from build123d import *

# Parameters (mm, degrees)
SKETCH_1_R          = 19.05
EXTRUDE_1_DEPTH     = 8
CUT_EXTRUDE_1_REACH = 53.347
SKETCH_2_R          = 2


with BuildPart() as part:
    # 스케치1 → 보스-돌출1 (new body)
    with BuildSketch(Plane.XY):
        with BuildLine():
            Line((-12.5, -18.708286934), (-12.5, -36.708286934))
            Line((-12.5, -36.708286934), (12.5, -36.708286934))
            Line((12.5, -36.708286934), (12.5, -18.708286934))
            ThreePointArc((12.5, -18.708286934), (0, 22.5), (-12.5, -18.708286934))
        make_face()
        Circle(SKETCH_1_R, mode=Mode.SUBTRACT)
    extrude(amount=EXTRUDE_1_DEPTH)

    # 스케치2 → 컷-돌출1 (cut, up to next)
    with BuildSketch(Plane.ZY.offset(12.5), mode=Mode.PRIVATE) as cut_extrude_1_sk1:
        with Locations(Location((4, -28.708286934, 0), (0, 0, 270))):
            Circle(SKETCH_2_R)
    cut_extrude_1_tool1 = extrude(cut_extrude_1_sk1.sketch, amount=-CUT_EXTRUDE_1_REACH, mode=Mode.PRIVATE) & part.part
    add(cut_extrude_1_tool1.solids().sort_by_distance((-12.5, -28.708287, 4))[0], mode=Mode.SUBTRACT)


solid = part.part
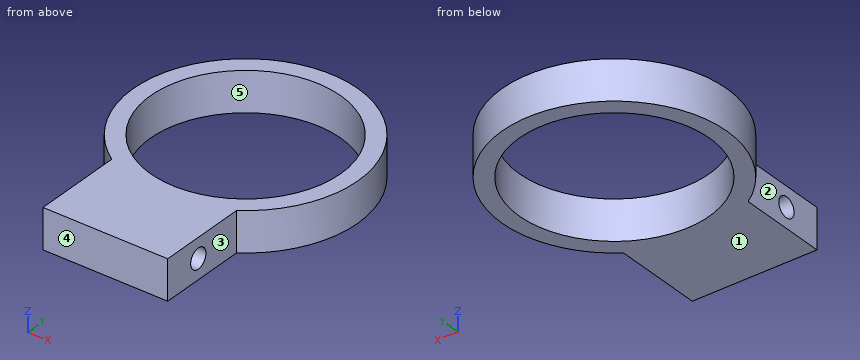
Geometry check sheet. Reference: the model listing, model coordinates, mm. Face numbers are marked on the shaded views. A direction names the side the tool comes from. Coordinates: 2 decimals unless noted, no trailing zeros. Loops run counter-clockwise (first coordinate to the right, second up) from the corner with the lowest first, then second, coordinate; pieces in that order, holes last. Notation, with made-up numbers: (79, 89) - (120, 89) arc R22 cw to (120, 122) - close; hole circle Ø9 at (71.5, 56.25). An arc over 180 degrees is marked (long way). Use one line per item in the form item = value. Start each with the question number.
Item 1: Section check B-B, the plane z = 4. Enter the section's corners in (x, y), and give its area (3 significant figures).
Item 2: Section check C-C, the plane x = -2. Enter the section's corners in (y, z).
Item 3: Section check D-D, the plane x = 16. Enter the section's corners in (y, z), and give its area (3 significant figures).
Item 4: Gauge pin test, flat ends, axial feed: pin 1 (8 mm diameter, centred on x = -12.5, y = -28, fed in from -Z); pin 2 (10 mm diameter, centred on x = -5, y = 8, fed in from -Z); pin 3 (4 mm diameter, centred on y = -27.5, z = 2.5, fed in from +X). Record the tip position at first contact, or that the pin passes through.
Item 5: Section check A-A, the plane y = 0. Enter the section's corners in (x, z).
Item 6: Tool access check on the marked faces 1 and 2. Record the directions out of +Z, -Z, +X, -X, +Y, -Y that give a thin tool (end or side, any length) a straight path to the whole face; none if there is none.
Item 7: Mould release check, pull along Y, two halves, no side actions. Record for the marked faces 3, 4 and 5: +Y half, -Y half, draft (parallel to the pull), parting line (faces both ways), or undercut.
Item 8: Thickness scan on probe 1 along Y at (x, z) = (-7.5, 3.5); probe 2 along Y at (x, z) = (-6.5, 2.5); probe 3 along Y at (x, z) = (10, 7). Record the ranges inside material, lowest first.
Computed:
q1.outline = (-12.5, -36.71) - (12.5, -36.71) - (12.5, -30.71) - (-12.5, -30.71) - close; (-12.5, -26.71) - (12.5, -26.71) - (12.5, -18.71) arc R22.5 ccw (long way) to (-12.5, -18.71) - close; hole circle Ø38.1 at (0, 0)
q1.area = 736 mm2
q2.outline = (-36.71, 0) - (-18.94, 0) - (-18.94, 8) - (-36.71, 8) - close; (18.94, 0) - (22.41, 0) - (22.41, 8) - (18.94, 8) - close; hole circle Ø4 at (-28.71, 4)
q3.outline = (-15.82, 0) - (-10.34, 0) - (-10.34, 8) - (-15.82, 8) - close; (10.34, 0) - (15.82, 0) - (15.82, 8) - (10.34, 8) - close
q3.area = 87.7 mm2
q4.pin_1 = 0
q4.pin_2 = through
q4.pin_3 = 12.5
q5.outline = (-22.5, 0) - (-19.05, 0) - (-19.05, 8) - (-22.5, 8) - close; (19.05, 0) - (22.5, 0) - (22.5, 8) - (19.05, 8) - close
q6.face_1 = -Z, +X, -X, +Y, -Y
q6.face_2 = +Z, -Z, -X, -Y
q7.face_3 = draft
q7.face_4 = -Y half
q7.face_5 = undercut
q8.probe_1 = -36.71 to -30.64, -26.77 to -17.51, 17.51 to 21.21
q8.probe_2 = -36.71 to -30.03, -27.39 to -17.91, 17.91 to 21.54
q8.probe_3 = -36.71 to -16.21, 16.21 to 20.16
